Autodesk Inventor part; units mm, degrees
ref_plane "Hex Key Sketch Plane" through (0, 0, 4.4) normal (0, 0, 1) x (1, 0, 0)
ref_plane "YZ Plane" through (0, 0, 0) normal (1, 0, 0) x (0, 1, 0)
ref_plane "XZ Plane" through (0, 0, 0) normal (0, 1, 0) x (-1, 0, 0)
sketch "Sketch1" plane through (0, 0, 0) normal (0, 0, 1) x (1, 0, 0)
  circle A0 centre (0, 0) radius 4
  dimension "Dia" = 8
extrude "Base" add sketch "Sketch1" against normal blind 18
ref_plane "Hex Key Sketch Plane" through (0, 0, 4.4) normal (0, 0, 1) x (1, 0, 0)
sketch "Sketch2" plane through (0, 0, 0) normal (0, 1, 0) x (-1, 0, 0)
  line L0 (0, -0.969) -> (0, 5.8139)
  line L1 (-4, 0) -> (4, 0)
  line L2 (0, 0) -> (7, 0)
  line L3 (7, 0) -> (7, 0.44)
  arc A0 (7, 0.44) -> (4.2, 4.4) centre (2.7997, 0.44) ccw
  line L4 (4.2, 4.4) -> (0, 4.4)
  line L5 (0, 4.4) -> (0, 0)
  dimension "d3" = 4.4
  dimension "d4" = 0.44
  dimension "d5" = 14
  dimension "d6" = 2.8
revolve "Button Head" add sketch "Sketch2" angle 360 about axis through (0, 0, -10) along (0, 0, 1)
sketch "Sketch4" plane through (0, 0, 0) normal (0, 1, 0) x (-1, 0, 0)
  line L0 (0, -0.88) -> (0, 5.28)
  line L1 (-4, 0) -> (4, 0)
  line L2 (0, 0) -> (7, 0)
  line L3 (7, 0) -> (7, 4.4)
  line L4 (7, 4.4) -> (0, 4.4)
  line L5 (0, 4.4) -> (0, 0)
  dimension "d13" = 4.4
  dimension "d14" = 14
revolve "Cap Head" [suppressed]
sketch "Sketch3" plane through (0, 0, 0) normal (0, 1, 0) x (-1, 0, 0)
  line L0 (0, -21.6) -> (0, 3.6)
  line L1 (-4, 0) -> (4, 0)
  line L2 (4, 0) -> (4, -18)
  line L3 (0, 0) -> (7, 0)
  line L4 (7, 0) -> (7, -0.44)
  line L5 (7, -0.44) -> (4, -4.4)
  line L6 (4, -4.4) -> (0, -4.4)
  line L7 (0, 0) -> (0, -4.4)
  dimension "d9" = 4.4
  dimension "d10" = 14
  dimension "d11" = 0.44
revolve "Flat Head" [suppressed]
sketch "Sketch5" plane through (0, 0, 4.4) normal (0, 0, 1) x (1, 0, 0)
  line L0 (1.4434, 2.5) -> (2.8868, 0)
  line L1 (2.8868, 0) -> (1.4434, -2.5)
  line L2 (1.4434, -2.5) -> (-1.4434, -2.5)
  line L3 (-1.4434, -2.5) -> (-2.8868, 0)
  line L4 (-2.8868, 0) -> (-1.4434, 2.5)
  line L5 (-1.4434, 2.5) -> (1.4434, 2.5)
  point P0 (0, 0)
  point P1 (0, 0)
  dimension "d16" = 5
extrude "Hex Socket" cut sketch "Sketch5" against normal blind 3.52
thread "Thread1"
equation "\"d3\" = H_K"
equation "\"d4\" = 0.1 * H_K"
equation "\"d5\" = Dk"
equation "\"d6\" = 0.2 * Dk"
equation "\"d13\" = H_K"
equation "\"d14\" = Dk"
equation "\"d9\" = H_K"
equation "\"d10\" = Dk"
equation "\"d11\" = 0.1 * H_K"
equation "\"d16\" = H_S"
equation "\"d17\" = 0.8 * H_K"
equation "\"Dk\" = 14"
equation "\"H_K\" = 4.4"
equation "\"H_S\" = 5"
equation "\"HexStartHeight\" = H_K"
properties part number "24-118-8" material "Steel, High Strength Low Alloy"
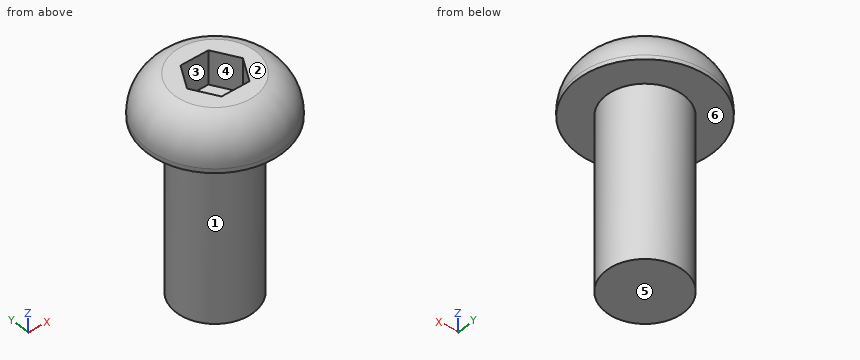
Read the model definition and answer for the solid it produces. Units are mm, in the model's axes. Face numbers are marked on the shaded views. A direction names the side the tool comes from. Give positions to 0.01 mm unless a question says otherwise; leave off trailing zeros. Write each loop counter-clockwise with the first axis right and the second up, starting at its lowest first coordinate (ties: lowest second). Pieces come first, ordered by that corner, then holes. Notation, with made-up numbers: (-14, 18.5) -> (29, 18.5) arc R24 ccw to (29, 42.5) -> close; hole circle Ø3 at (55, -30). An arc over 180 degrees is marked (long way). Answer in a Markdown table with one row per item.
1) Determine the mould class of the marked faces 1, 2, 3 and 4 for opening direction Y: released by +Y, released by -Y, zero draft, split by the parting line, or undercut.
Results list:
| item | result |
|---|---|
| face 1 | split by the parting line |
| face 2 | zero draft |
| face 3 | undercut |
| face 4 | undercut |
2) A tool of negligible diameter and unlimited length cuts with its end or side. For the marked faces 5 and 6, from which of +Z, -Z, +X, -X, +Y, -Y can it reach the whole face along a straight path? Write none if from no direction.
Results list:
| item | result |
|---|---|
| face 5 | -Z, +X, -X, +Y, -Y |
| face 6 | -Z |
3) Each of these flat-tipped pins is pushed along its axis until it touches: pin 1 Ø1.5 at (x, z) = (-5, -7.5) entering from -Y; pin 2 Ø3 at (x, z) = (0.5, 2.5) entering from +Y; pin 3 Ø1.5 at (x, y) = (0, -0.5) entering from +Z; pin 4 Ø3 at (x, z) = (-3.5, -13) entering from -Y. Where does it stop, or does it pass through?
Results list:
| item | result |
|---|---|
| pin 1 | through |
| pin 2 | y = 6.96 |
| pin 3 | z = 0.88 |
| pin 4 | y = -3.46 |
4) Section A-A on z = -4.25 is taken. Give the vertices of the cut face in (x, y), plus the area to 3 significant figures.
Results list:
| item | result |
|---|---|
| outline | circle Ø8 at (0, 0) |
| area | 50.3 mm^2 |
5) Straight lines are drawn through the part: line 1 (Z direction, x = 4, y = 4.75); line 2 (Y direction, x = 2.25, z = 2.5); line 3 (Z direction, x = -1.5, y = 0.75). For each, find the intervals that lie inside material, in ascending order. Write a range as [from, to].
Results list:
| item | result |
|---|---|
| line 1 | [0, 2.89] |
| line 2 | [-6.06, -1.1], [1.1, 6.06] |
| line 3 | [-18, 0.88] |
